from build123d import *

# Parameters (mm, degrees)
SKETCH1_R           = 2.75
BOSS_EXTRUDE1_DEPTH = 35
SKETCH2_R           = 2.75
BOSS_EXTRUDE2_DEPTH = 35


with BuildPart() as part:
    # Sketch1 → Boss-Extrude1 (new body)
    with BuildSketch(Plane(origin=(0, 0, 0), x_dir=(1, 0, 0), z_dir=(0, 1, 0))):
        with BuildLine():
            Line((7.5, 44.72), (7.5, 0))
            ThreePointArc((7.5, 0), (0, -7.5), (-7.5, 0))
            Line((-7.5, 0), (-7.5, 44.72))
            ThreePointArc((-7.5, 44.72), (0, 52.22), (7.5, 44.72))
        make_face()
        with Locations((0, 44.72)):
            Circle(SKETCH1_R, mode=Mode.SUBTRACT)
        Circle(SKETCH1_R, mode=Mode.SUBTRACT)
    extrude(amount=BOSS_EXTRUDE1_DEPTH)

    # Sketch2 → Boss-Extrude2 (add)
    with BuildSketch(Plane.XZ):
        with BuildLine():
            ThreePointArc((-75.875539691, 60.413455223), (-95.106545537, 57.577650686), (-95.38977649, 38.140748838))
            Line((-95.38977649, 38.140748838), (-19.065447836, -54.271984943))
            ThreePointArc((-19.065447836, -54.271984943), (2.051984943, -56.285447836), (4.065447836, -35.168015057))
            Line((4.065447836, -35.168015057), (-13.698799918, -13.659241545))
            ThreePointArc((-13.698799918, -13.659241545), (5.718972245, -7.089342197), (0.448788963, 12.720721442))
            Line((0.448788963, 12.720721442), (-75.875539691, 60.413455223))
        make_face()
        Circle(SKETCH2_R, mode=Mode.SUBTRACT)
        with Locations((0, -44.72)):
            Circle(SKETCH2_R, mode=Mode.SUBTRACT)
    extrude(amount=-BOSS_EXTRUDE2_DEPTH)


solid = part.part
Geometry check sheet. Reference: the model listing, model coordinates, mm. Round coordinates to 2 decimals unless told otherwise and drop trailing zeros. Order: outer loops, then holes, each group sorted by start corner. A loop starts at its lowest first (then second) coordinate and runs counter-clockwise, first axis right, second up. Notation, with made-up numbers: M -26,85.5 L -13,85.5 A11 cw -13,103.5 Z; hole C 57.5,19.5 d9. An arc over 180 degrees is marked long. Answer in a Markdown table with one row per item.
(1) Scan lines: probe 1 along Z at (x, y) = (0, 10); probe 2 along Z at (x, y) = (2.5, 16); probe 3 along X at (y, z) = (16, -44.72). Record each from-to range of solid material in increasing order. Write a range as from..to.
Responses:
| item | result |
|---|---|
| probe 1 | z = -57.71..-47.47, -41.97..-2.75, 2.75..13 |
| probe 2 | z = -55.9..-45.87, -43.57..-1.15, 1.15..11.18 |
| probe 3 | x = -26.95..-2.75, 2.75..7.5 |
(2) Draft check along X on faces 1 (the face through (5.67, 17.26, 7.18)), 2 (the face through (-94.91, 17.26, 57.8)), 3 (the face through (-35, 35, 2)), 4 (the face through (-0.596, 17.255, -42.035)). Enter one of: released by +X, released by -X, zero draft, split by the parting line, or undercut.
Responses:
| item | result |
|---|---|
| face 1 | released by +X |
| face 2 | split by the parting line |
| face 3 | zero draft |
| face 4 | undercut |
(3) Sectioned sample at C-C, the plane z = -6. Record the cut outline in (x, y).
Responses:
| item | result |
|---|---|
| outline | M -58.93,0 L 7.5,0 L 7.5,35 L -58.93,35 Z |
(4) Sectioned sample at A-A, the plane y = 32.5. Record the cut outline in (x, z), and give its area (3 significant figures).
Responses:
| item | result |
|---|---|
| outline | M -95.39,38.14 L -19.07,-54.27 A15 ccw 7.5,-44.72 L 7.5,0 A15 ccw 0.45,12.72 L -75.88,60.41 A15 ccw Z; hole M -13.7,-13.66 L -7.5,-21.16 L -7.5,-15 A15 cw Z; hole C 0,-44.72 d5.5; hole C 0,0 d5.5 |
| area | 6,170 mm² |
(5) Go/stop test with flat-tipped pins: P1, Ø12, axis at x = -34, y = 22, coming from the +Z side; P2, Ø10, axis at y = 13.5, z = -29, coming from the -X side; P3, Ø6, axis at x = -55.5, y = 26.5, coming from the -Z side. Record where each tip stops, or that it passes through.
Responses:
| item | result |
|---|---|
| P1 | stops at z = 38 |
| P2 | stops at x = -44.07 |
| P3 | stops at z = -13.79 |
(6) Sectioned sample at B-B, the plane x = -42. Record the cut outline in (y, z), and give its area (3 significant figures).
Responses:
| item | result |
|---|---|
| outline | M 0,-26.5 L 35,-26.5 L 35,39.25 L 0,39.25 Z |
| area | 2,300 mm² |
